For this review, take the finished solid that the model builds, in its own axes (mm). Face numbers are marked on the shaded views. A direction names the side the tool comes from. Round coordinates to 2 decimals unless told otherwise and drop trailing zeros. Loops run counter-clockwise (first coordinate to the right, second up) from the corner with the lowest first, then second, coordinate; pieces in that order, holes last. Notation, with made-up numbers: (-23.5, -18.75) -> (2.5, -18.75) arc R31 ccw to (2.5, 19.25) -> close; hole circle Ø11 at (-7, -34). An arc over 180 degrees is marked (long way). Use one line per item in the form item = value. Start each with the question number.
from build123d import *

# Parameters (mm, degrees)
F1_DEPTH = 3
F2_R     = 3
F3_DEPTH = 3
F5_DEPTH = 41
F6_R     = 1.25
F7_R     = 3
F8_DEPTH = 3


with BuildPart() as f1:
    # F0 (on Top) → F1 (new body)
    with BuildSketch(Plane.XY):
        with BuildLine():
            ThreePointArc((3.4900408275, -3.4019155104), (0, -1.9823645076), (-3.4900408275, -3.4019155104))
            Line((-3.4900408275, -3.4019155104), (-19.7450204138, -19.2464485424))
            ThreePointArc((-19.7450204138, -19.2464485424), (-20.3035354387, -20.065218213), (-20.5, -21.036673041))
            Line((-20.5, -21.036673041), (-20.5, -22.9823645076))
            Line((-20.5, -22.9823645076), (20.5, -22.9823645076))
            Line((20.5, -22.9823645076), (20.5, -21.036673041))
            ThreePointArc((20.5, -21.036673041), (20.3035354387, -20.065218213), (19.7450204138, -19.2464485424))
            Line((19.7450204138, -19.2464485424), (3.4900408275, -3.4019155104))
        make_face()
    extrude(amount=F1_DEPTH)

    # F2 (on face) → F3 (cut)
    with BuildSketch(Plane.XY.offset(3)):
        with Locations((0, -11.9823645076)):
            Circle(F2_R)
    extrude(amount=-F3_DEPTH, mode=Mode.SUBTRACT)

    # F4 (on face) → F5 (join)
    with BuildSketch(Plane(origin=(-20.5, 0, 0), x_dir=(0, -1, 0), z_dir=(-1, 0, 0))):
        with BuildLine():
            Line((31.0350133065, 10.4936538032), (22.9823645076, 3))
            Line((22.9823645076, 3), (22.9823645076, 0))
            Line((22.9823645076, 0), (23.1790209905, 0))
            ThreePointArc((23.1790209905, 0), (24.0940705422, 0.1734823624), (24.8821241276, 0.6698525457))
            Line((24.8821241276, 0.6698525457), (33.078737071, 8.2974768581))
            Line((33.078737071, 8.2974768581), (31.0350133065, 10.4936538032))
        make_face()
    extrude(amount=-F5_DEPTH)

    # F6
    f6_edges = [f1.edges().sort_by_distance(p)[0] for p in [
        (0, -22.982365, 3),
    ]]
    fillet(f6_edges, radius=F6_R)

    # F7 (on face) → F8 (cut)
    with BuildSketch(Plane(origin=(0, -9.1697511003, -9.8537758913), x_dir=(1, 0, 0), z_dir=(0, 0.6812412548, 0.7320589817))):
        with Locations((13.5, -23.3598113305)):
            Circle(F7_R)
        with Locations((0, -23.3598113305)):
            Circle(F7_R)
        with Locations((-13.5, -23.3598113305)):
            Circle(F7_R)
    extrude(amount=-F8_DEPTH, mode=Mode.SUBTRACT)


solid = f1.part
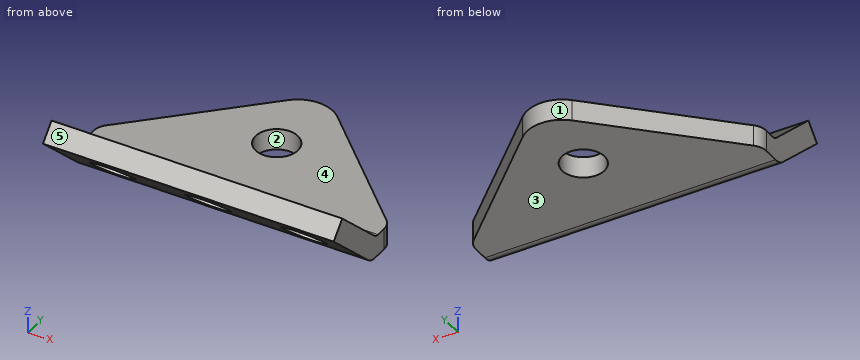
Item 1: Draft analysis for pull direction Y (two halves, no side actions). For the marked faces 1, 2 and 3, state which applies: +Y half, -Y half, draft (parallel to the pull), parting line (faces both ways), or undercut.
Item 2: Take a section at A-A on y = -11. Give the boundary of the cut face in (x, z).
Item 3: Machinability: for the marked faces 4 and 5, which of the approach directions +Z, -Z, +X, -X, +Y, -Y give a long, thin tool a straight path to every point of the face, cutting with its end or side? Answer none if there is none.
Item 4: For P1, Ø2, axis at x = -12, z = 2, coming from the +Y side; P2, Ø1, axis at x = 11, z = 1, coming from the +Y side; P3, Ø6, axis at x = -12.5, z = 7, coming from the -Y side, all flat-tipped, find the tip position at first contact; note any pin that passes through.
Item 5: Take a section at D-D on x = 5. Give the boundary of the cut face in (y, z).
Item 6: Wall thickness on line 1 (Z direction, x = 16.5, y = -19.5); line 2 (Y direction, x = 0, z = 1.25); line 3 (X direction, y = -26, z = 3.25): over which ranges is each line inside the solid? List them lowest first.
Item 7: Take a section at B-B on x = 0. Give the boundary of the cut face in (y, z).
Item 8: Take a section at C-C on x = -18. Give the boundary of the cut face in (y, z), plus the area to 3 significant figures.
Results:
q1.face_1 = +Y half
q1.face_2 = undercut
q1.face_3 = draft
q2.outline = (-11.28, 0) -> (-2.83, 0) -> (-2.83, 3) -> (-11.28, 3) -> close; (2.83, 0) -> (11.28, 0) -> (11.28, 3) -> (2.83, 3) -> close
q3.face_4 = +Z, +X, -X, +Y
q3.face_5 = +Z, +X, -X, -Y
q4.P1 = -10.72
q4.P2 = -10.23
q4.P3 = -33.08
q5.outline = (-33.08, 8.3) -> (-24.88, 0.67) arc R2.5 ccw to (-23.18, 0) -> (-4.87, 0) -> (-4.87, 3) -> (-22.49, 3) arc R1.25 cw to (-23.34, 3.33) -> (-31.04, 10.49) -> close
q6.line_1 = 0 to 3
q6.line_2 = -25.51 to -14.98, -8.98 to -1.98
q6.line_3 = -20.5 to -15.63, -11.37 to -2.13, 2.13 to 11.37, 15.63 to 20.5
q7.outline = (-33.08, 8.3) -> (-30.51, 5.91) -> (-28.47, 8.1) -> (-31.04, 10.49) -> close; (-26.12, 1.82) -> (-24.88, 0.67) arc R2.5 ccw to (-23.18, 0) -> (-14.98, 0) -> (-14.98, 3) -> (-22.49, 3) arc R1.25 cw to (-23.34, 3.33) -> (-24.07, 4.02) -> close; (-8.98, 0) -> (-1.98, 0) -> (-1.98, 3) -> (-8.98, 3) -> close
q8.outline = (-33.08, 8.3) -> (-24.88, 0.67) arc R2.5 ccw to (-23.18, 0) -> (-17.55, 0) -> (-17.55, 3) -> (-22.49, 3) arc R1.25 cw to (-23.34, 3.33) -> (-31.04, 10.49) -> close
q8.area = 52.8 mm2
